```python
from build123d import *

# Parameters (mm, degrees)
SKETCH1_W           = 50.8
SKETCH1_H           = 12.7
BOSS_EXTRUDE1_DEPTH = 12.7
SKETCH2_R           = 3.429
CUT_EXTRUDE1_DEPTH  = 32.108519733
CUT_EXTRUDE2_DEPTH  = 2.794


with BuildPart() as part:
    # Sketch1 → Boss-Extrude1 (new body)
    with BuildSketch(Plane(origin=(0, 0, 0), x_dir=(1, 0, 0), z_dir=(0, 1, 0))):
        with Locations((0, 6.35)):
            Rectangle(SKETCH1_W, SKETCH1_H)
    extrude(amount=BOSS_EXTRUDE1_DEPTH)

    # Sketch2 → Cut-Extrude1 (cut, through all)
    with BuildSketch(Plane(origin=(0, 12.7, 0), x_dir=(1, 0, 0), z_dir=(0, 1, 0))):
        with Locations(Location((-19.05, 6.35, 0), (0, 0, 270))):
            Circle(SKETCH2_R)
        with Locations(Location((19.05, 6.35, 0), (0, 0, 270))):
            Circle(SKETCH2_R)
        with Locations(Location((0, 6.35, 0), (0, 0, 270))):
            Circle(SKETCH2_R)
    extrude(amount=-CUT_EXTRUDE1_DEPTH, mode=Mode.SUBTRACT)

    # Sketch3 → Cut-Extrude2 (cut, symmetric)
    with BuildSketch(Plane(origin=(0, 6.35, 0), x_dir=(1, 0, 0), z_dir=(0, 1, 0))):
        Polygon((-6.30581964, 6.35), (-6.30581964, 19.396139052), (6.30581964, 19.396139052), (6.30581964, 6.35), (3.15290982, 0.889), (-3.15290982, 0.889), align=None)
    extrude(amount=CUT_EXTRUDE2_DEPTH, both=True, mode=Mode.SUBTRACT)


solid = part.part
```
Could you check a few things on this model? Use its own coordinates, in mm. A direction names the side the tool comes from. Give positions to 0.01 mm unless a question says otherwise; leave off trailing zeros. Order: outer loops, then holes, each group sorted by start corner. A loop starts at its lowest first (then second) coordinate and runs counter-clockwise, first axis right, second up.
Q1. Suppose I cut it at D-D, the plane y = 1.25. Write out the boundary of the cut face in (x, z).
Q2. I'm going to push flat-ended pins straight in: P1, Ø5.5, axis at x = -19.05, z = -6.35, coming from the -Y side; P2, Ø1.7, axis at x = -1, y = 6, coming from the -Z side. Where does each tip first touch, or does it pass through?
Q3. If I drill on line 1 along X through (y, z) = (1.45, -6.35); line 2 along X through (y, z) = (7.5, -6.35); line 3 along Y through (x, z) = (-4.5, -7.75), over which ranges is the centre line in solid material (lowest first)?
Q4. For faces 4 (the cylindrical face through (-1.31, 1.8, -3.18)), 5 (the flat face through (0, 6, -0.889)), which set-ups out of +Z, -Z, +X, -X, +Y, -Y let a thin tool reach every point of the face, with its end or its side?
Q5. We'd pull the mould along X, two halves only. Please class faces 1 (the flat face through (6.306, 6, -10)), 2 (the flat face through (0, 6, 0)), 3 (the flat face through (25.4, 6, -6)): +X half, -X half, draft (parallel to the pull), parting line (faces both ways), or undercut.
Q6. Suppose I cut it at A-A, the plane x = 19.05. Write out the boundary of the cut face in (y, z), and give its area (3 significant figures).
Q7. Suppose I cut it at C-C, the plane z = -5.25. Write out the boundary of the cut face in (x, y), and give its area (3 significant figures).
Q8. Suppose I cut it at B-B, the plane x = 0. Write out the boundary of the cut face in (y, z).
Solution:
1. outline: (-25.4, -12.7) - (25.4, -12.7) - (25.4, 0) - (-25.4, 0) - close; hole circle Ø6.86 at (-19.05, -6.35); hole circle Ø6.86 at (0, -6.35); hole circle Ø6.86 at (19.05, -6.35)
2. P1: passes through
2. P2: stops at z = -0.89
3. line 1: x = -25.4 to -22.48, -15.62 to -3.43, 3.43 to 15.62, 22.48 to 25.4
3. line 2: x = -25.4 to -22.48, -15.62 to -6.31, 6.31 to 15.62, 22.48 to 25.4
3. line 3: y = 0 to 3.56, 9.14 to 12.7
4. face 4: +Y, -Y
4. face 5: -Z
5. face 1: undercut
5. face 2: draft
5. face 3: +X half
6. outline: (0, -12.7) - (12.7, -12.7) - (12.7, -9.78) - (0, -9.78) - close; (0, -2.92) - (12.7, -2.92) - (12.7, 0) - (0, 0) - close
6. area: 74.2 mm2
7. outline: (-25.4, 0) - (-22.3, 0) - (-22.3, 12.7) - (-25.4, 12.7) - close; (-15.8, 0) - (-3.25, 0) - (-3.25, 3.56) - (-5.67, 3.56) - (-5.67, 9.14) - (-3.25, 9.14) - (-3.25, 12.7) - (-15.8, 12.7) - close; (3.25, 0) - (15.8, 0) - (15.8, 12.7) - (3.25, 12.7) - (3.25, 9.14) - (5.67, 9.14) - (5.67, 3.56) - (3.25, 3.56) - close; (22.3, 0) - (25.4, 0) - (25.4, 12.7) - (22.3, 12.7) - close
7. area: 371 mm2
8. outline: (0, -12.7) - (3.56, -12.7) - (3.56, -9.78) - (0, -9.78) - close; (0, -2.92) - (3.56, -2.92) - (3.56, -0.89) - (9.14, -0.89) - (9.14, -2.92) - (12.7, -2.92) - (12.7, 0) - (0, 0) - close; (9.14, -12.7) - (12.7, -12.7) - (12.7, -9.78) - (9.14, -9.78) - close
